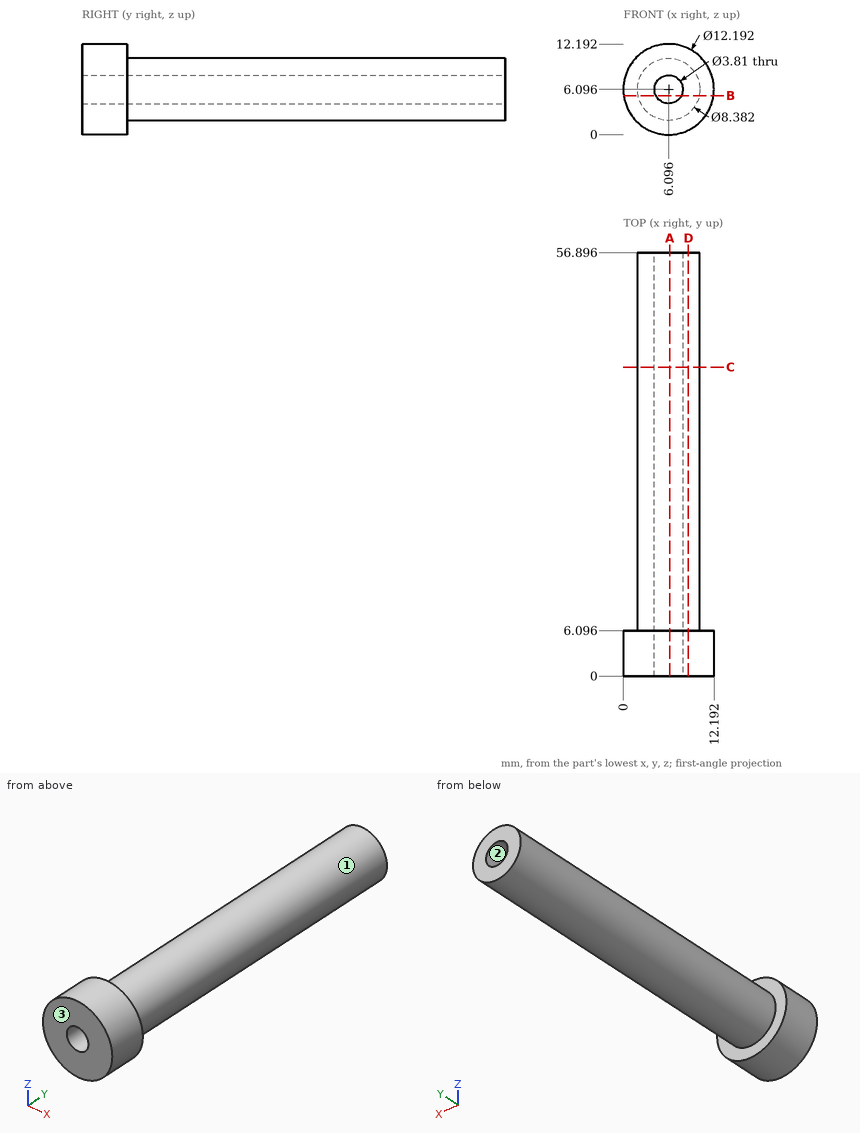
Can you work these out from the drawing? Everything is in mm from the part's minimum corner. Give positions to 0.01 mm unless a question says otherwise; leave off trailing zeros. Loops run counter-clockwise (first coordinate to the right, second up) from the corner with the lowest first, then second, coordinate; pieces in that order, holes last. Notation, with made-up numbers: (38, 29) -> (61, 29) arc R35 ccw to (61, 65) -> close; hole circle Ø1 at (-1.75, 11). An arc over 180 degrees is marked (long way). Return JSON: item names as keys, results as strings.
Item 1: If we section it at C-C on y = 41.5: List the corners of the cut face in (x, z) for me (3 decimals), plus the area to 3 significant figures.
Geometry results:
{"outline": "circle Ø8.382 at (6.096, 6.096); hole circle Ø3.81 at (6.096, 6.096)", "area": "43.8 mm²"}
Item 2: We'd pull the mould along X, two halves only. Please class the marked faces 1, 2 and 3: +X half, -X half, draft (parallel to the pull), parting line (faces both ways), or undercut.
Geometry results:
{"face 1": "parting line", "face 2": "undercut", "face 3": "draft"}
Item 3: If we section it at D-D on x = 8.75: List the corners of the cut face in (y, z) for me, plus the area to 3 significant figures.
Geometry results:
{"outline": "(0, 0.61) -> (6.1, 0.61) -> (6.1, 2.85) -> (56.9, 2.85) -> (56.9, 9.34) -> (6.1, 9.34) -> (6.1, 11.58) -> (0, 11.58) -> close", "area": "396 mm²"}
Item 4: If we section it at B-B on z = 5.25: List the corners of the cut face in (x, y) for me.
Geometry results:
{"outline": "(0.06, 0) -> (4.39, 0) -> (4.39, 56.9) -> (1.99, 56.9) -> (1.99, 6.1) -> (0.06, 6.1) -> close; (7.8, 0) -> (12.13, 0) -> (12.13, 6.1) -> (10.2, 6.1) -> (10.2, 56.9) -> (7.8, 56.9) -> close"}
Item 5: I'm going to push flat-ended pins straight in: pin 1 (4 mm diameter, centred on y = 12, z = 1.5, fed in from -X); pin 2 (6 mm diameter, centred on x = 6, y = 39, fed in from +Z); pin 3 (2 mm diameter, centred on x = 7.5, y = 9, fed in from -Z). Where does each tip first touch, or does it pass through?
Geometry results:
{"pin 1": "stops at x = 2.81", "pin 2": "stops at z = 10.29", "pin 3": "stops at z = 1.92"}
Item 6: I need wall thicknesses on L1, parallel to X at y = 25, z = 6.25; L2, parallel to Z at x = 7, y = 51.5; L3, parallel to Y at x = 10.25, z = 2.5. Which ranges of each line are inside material? Lowest first, please. Write a range as from..to.
Geometry results:
{"L1": "x = 1.91..4.2, 7.99..10.28", "L2": "z = 2..4.42, 7.77..10.19", "L3": "y = 0..6.1"}
Item 7: If we section it at A-A on x = 6.25: List the corners of the cut face in (y, z) for me.
Geometry results:
{"outline": "(0, 0) -> (6.1, 0) -> (6.1, 1.91) -> (56.9, 1.91) -> (56.9, 4.2) -> (0, 4.2) -> close; (0, 7.99) -> (56.9, 7.99) -> (56.9, 10.28) -> (6.1, 10.28) -> (6.1, 12.19) -> (0, 12.19) -> close"}
